Geometry check sheet. Reference: the model listing, model coordinates, mm. Face numbers are marked on the shaded views. A direction names the side the tool comes from. Give positions to 0.01 mm unless a question says otherwise; leave off trailing zeros. Write each loop counter-clockwise with the first axis right and the second up, starting at its lowest first coordinate (ties: lowest second). Pieces come first, ordered by that corner, then holes. Notation, with made-up numbers: (-12, 19) -> (31, 19) arc R37 cw to (31, 58) -> close; hole circle Ø8 at (36.25, -8.5). An arc over 180 degrees is marked (long way). Use a Markdown table: item, result. Add a question column.
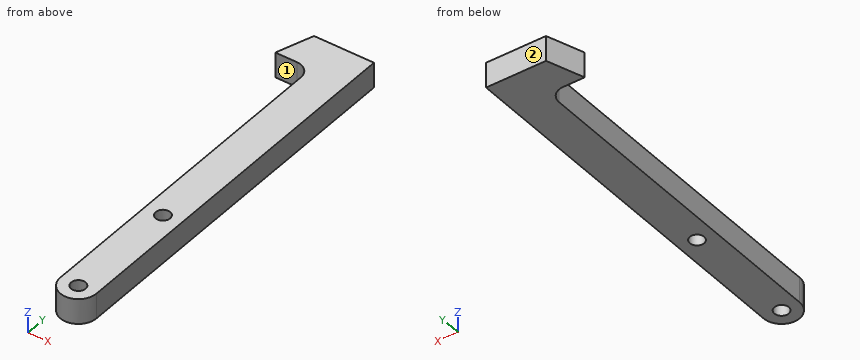
from build123d import *

# Parameters (mm, degrees)
BOSS_EXTRU_1_DEPTH      = 3.5
ESQUISSE3_R             = 1
ENL_V_MAT_EXTRU_1_DEPTH = 4
ESQUISSE4_R             = 1
ENL_V_MAT_EXTRU_2_DEPTH = 10
ENL_V_MAT_EXTRU_3_DEPTH = 57.011159602
CONG_1_R                = 2


with BuildPart() as part:
    # Esquisse1 → Boss.-Extru.1 (new body)
    with BuildSketch(Plane.XY):
        with BuildLine():
            Line((0, 0), (10, 0))
            Line((10, 0), (10, -52.5))
            ThreePointArc((10, -52.5), (7.5, -55), (5, -52.5))
            Line((5, -52.5), (5, -5))
            Line((5, -5), (0, -5))
            Line((0, -5), (0, 0))
        make_face()
    extrude(amount=BOSS_EXTRU_1_DEPTH)

    # Esquisse3 → Enlèv. mat.-Extru.1 (cut)
    with BuildSketch(Plane(origin=(0, 0, 0), x_dir=(-1, 0, 0), z_dir=(0, 0, -1))):
        with Locations((-7.5, -52.5)):
            Circle(ESQUISSE3_R)
    extrude(amount=-ENL_V_MAT_EXTRU_1_DEPTH, mode=Mode.SUBTRACT)

    # Esquisse4 → Enlèv. mat.-Extru.2 (cut)
    with BuildSketch(Plane.XY.offset(3.5)):
        with Locations((7.5, -36.5)):
            Circle(ESQUISSE4_R)
    extrude(amount=-ENL_V_MAT_EXTRU_2_DEPTH, mode=Mode.SUBTRACT)

    # Esquisse5 → Enlèv. mat.-Extru.3 (cut, through all)
    with BuildSketch(Plane.XY.offset(3.5)):
        Polygon((0, 0), (1.700931961, 0), (0, -5), align=None)
    extrude(amount=-ENL_V_MAT_EXTRU_3_DEPTH, mode=Mode.SUBTRACT)

    # Congé1
    cong_1_edges = [part.edges().sort_by_distance(p)[0] for p in [
        (5, -5, 1.75),
    ]]
    fillet(cong_1_edges, radius=CONG_1_R)


solid = part.part
1) Sectioned sample at C-C, the plane z = 2.65. Enter the section's corners in (x, y), and give its area (3 significant figures).
2) Sectioned sample at A-A, the plane y = -36.5. Enter the section's corners in (x, z).
3) Material ranges on probe 1 along Y at (x, z) = (7.5, 2); probe 2 along X at (y, z) = (-22, 3.2); probe 3 along Y at (x, z) = (9.75, 2.9), recorded low to high. Write a range as [from, to].
4) Sectioned sample at B-B, the plane x = 7.5. Enter the section's corners in (y, z), and give its area (4 significant figures).
5) Sectioned sample at D-D, the plane y = -13.5. Enter the section's corners in (x, z).
6) Tool access check on the marked faces 1 and 2. Record the directions out of +Z, -Z, +X, -X, +Y, -Y that give a thin tool (end or side, any length) a straight path to the whole face; none if there is none.
7) Gauge pin test, flat ends, axial feed: P1, Ø1.8, axis at x = 7.5, y = -36.5, coming from the +Z side; P2, Ø0.9, axis at x = 1.5, z = 2, coming from the -Y side; P3, Ø1.5, axis at x = 9, z = 2, coming from the -Y side. Record the tip position at first contact, or that the pin passes through.
Check values:
| question | item | result |
|---|---|---|
| 1 | outline | (0, -5) -> (3, -5) arc R2 cw to (5, -7) -> (5, -52.5) arc R2.5 ccw to (10, -52.5) -> (10, 0) -> (1.7, 0) -> close; hole circle Ø2 at (7.5, -52.5); hole circle Ø2 at (7.5, -36.5) |
| 1 | area | 288 mm² |
| 2 | outline | (5, 0) -> (6.5, 0) -> (6.5, 3.5) -> (5, 3.5) -> close; (8.5, 0) -> (10, 0) -> (10, 3.5) -> (8.5, 3.5) -> close |
| 3 | probe 1 | [-55, -53.5], [-51.5, -37.5], [-35.5, 0] |
| 3 | probe 2 | [5, 10] |
| 3 | probe 3 | [-53.59, 0] |
| 4 | outline | (-55, 0) -> (-53.5, 0) -> (-53.5, 3.5) -> (-55, 3.5) -> close; (-51.5, 0) -> (-37.5, 0) -> (-37.5, 3.5) -> (-51.5, 3.5) -> close; (-35.5, 0) -> (0, 0) -> (0, 3.5) -> (-35.5, 3.5) -> close |
| 4 | area | 178.5 mm² |
| 5 | outline | (5, 0) -> (10, 0) -> (10, 3.5) -> (5, 3.5) -> close |
| 6 | face 1 | +Z, -Z, -X, -Y |
| 6 | face 2 | +Z, -Z, +X, -X, +Y |
| 7 | P1 | through |
| 7 | P2 | y = -5 |
| 7 | P3 | y = -54.88 |
